Check sheet for the modelled part. Datum: model origin and axes. Units: mm. Face numbers are marked on the shaded views. A direction names the side the tool comes from. Give positions to 0.01 mm unless a question says otherwise; leave off trailing zeros. Write each loop counter-clockwise with the first axis right and the second up, starting at its lowest first coordinate (ties: lowest second). Pieces come first, ordered by that corner, then holes. Notation, with made-up numbers: (16, 37) -> (47, 37) arc R22 ccw to (47, 56) -> close; hole circle Ø4 at (-5, 68). An arc over 180 degrees is marked (long way). Use a Markdown table: item, result. Add a question column.
1. Cross-section at A-A (z = -140). Enter the section's corners in (x, y), then the cut area to 3 significant figures.
2. Set-up check for the marked faces 1 and 2: record each of +Z, -Z, +X, -X, +Y, -Y from which the full face is reachable in a straight line by a thin tool's end or side.
3. Cross-section at C-C (y = 2.5). Enter the section's corners in (x, z).
4. Cross-section at B-B (x = -150.5). Enter the section's corners in (y, z), then the cut area to 3 significant figures.
5. Release check for a two-part mould opening along Y. For the marked faces 3, 4 and 5 record: released by +Y, released by -Y, zero draft, split by the parting line, or undercut.
6. Scan lines: probe 1 along X at (y, z) = (38, 58.5); probe 2 along Y at (x, z) = (57.5, -215); probe 3 along Z at (x, y) = (170, 239.5). Record each from-to range of solid material in increasing order. Write a range as [from, to].
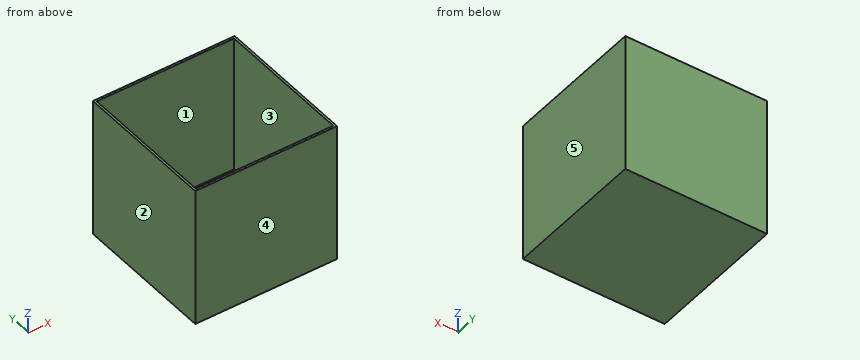
from build123d import *

# Parameters (mm, degrees)
F0_W     = 800
F0_H     = 800
F1_DEPTH = 400
F2_T     = -12.7
F3_W     = 1.108050679
F3_H     = 800
F3_W_2   = 798.891949321
F4_DEPTH = 12.7


with BuildPart() as f1:
    # F0 (on Front) → F1 (new body, symmetric)
    with BuildSketch(Plane.XZ):
        with Locations((67.3246156823, 84.0211848542)):
            Rectangle(F0_W, F0_H)
    extrude(amount=F1_DEPTH, both=True)

    # F2 (hollow: no face is removed)
    offset(amount=F2_T, mode=Mode.SUBTRACT)

    # F3 (on face) → F4 (cut)
    with BuildSketch(Plane.XY.offset(484.0211848542)):
        with Locations((-332.1213589782, 0)):
            Rectangle(F3_W, F3_H)
        with Locations((67.8786410218, 0)):
            Rectangle(F3_W_2, F3_H)
    extrude(amount=-F4_DEPTH, mode=Mode.SUBTRACT)


solid = f1.part
Worked answers:
| question | item | result |
|---|---|---|
| 1 | outline | (-332.68, -400) -> (467.32, -400) -> (467.32, 400) -> (-332.68, 400) -> close; hole (-319.98, -387.3) -> (454.62, -387.3) -> (454.62, 387.3) -> (-319.98, 387.3) -> close |
| 1 | area | 40,000 mm² |
| 2 | face 1 | +Z |
| 2 | face 2 | +Z, -Z, -X, +Y, -Y |
| 3 | outline | (-332.68, -315.98) -> (467.32, -315.98) -> (467.32, 471.32) -> (454.62, 471.32) -> (454.62, -303.28) -> (-319.98, -303.28) -> (-319.98, 471.32) -> (-332.68, 471.32) -> close |
| 4 | outline | (-400, -315.98) -> (400, -315.98) -> (400, 471.32) -> (387.3, 471.32) -> (387.3, -303.28) -> (-387.3, -303.28) -> (-387.3, 471.32) -> (-400, 471.32) -> close |
| 4 | area | 29,800 mm² |
| 5 | face 3 | undercut |
| 5 | face 4 | released by -Y |
| 5 | face 5 | zero draft |
| 6 | probe 1 | x = [-332.68, -319.98], [454.62, 467.32] |
| 6 | probe 2 | y = [-400, -387.3], [387.3, 400] |
| 6 | probe 3 | z = [-315.98, -303.28] |
